Part model, mm, in its own coordinate system. Face numbers are marked on the shaded views. Coordinates: 2 decimals unless noted, no trailing zeros. Order: outer loops, then holes, each group sorted by start corner. A loop starts at its lowest first (then second) coordinate and runs counter-clockwise, first axis right, second up.
1) Mould opens along Z. For the marked faces 1, 2 and 3 say: +Z half, -Z half, draft (parallel to the pull), parting line (faces both ways), or undercut.
2) Cut at B-B (z = 11.25). List the corners of the cut face in (x, y), and give its area (3 significant figures).
3) Wall check: L1, parallel to Y at x = 8.3, z = 0.5; L2, parallel to Z at x = 8.75, y = 6.75; L3, parallel to Y at x = 7, z = 1.75. Give the ranges that are in metal, low to high.
4) Cut at C-C (y = 0). List the corners of the cut face in (x, z).
5) Cut at A-A (x = 8.3). List the corners of the cut face in (y, z).
6) Pin check, flat tips, straight feed: pin 1 Ø5 at (y, z) = (5.5, 2.5) entering from +X; pin 2 Ø0.5 at (y, z) = (4.5, 7) entering from +X; pin 3 Ø2 at (x, z) = (8, 3.5) entering from +Y; pin 4 Ø4.5 at (x, z) = (7.5, 5.5) entering from -Y. Stop position of each tip, or through.
7) Cut at D-D (x = 4.25). List the corners of the cut face in (y, z).
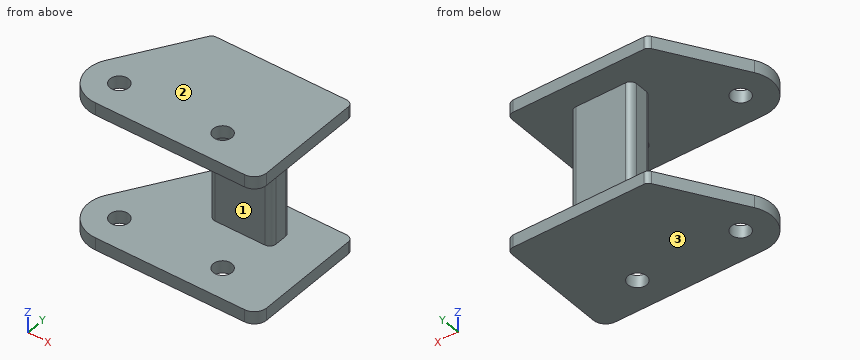
```python
from build123d import *

# Parameters (mm, degrees)
SKETCH1_R           = 0.75
BOSS_EXTRUDE1_DEPTH = 1
BOSS_EXTRUDE2_START = 1
BOSS_EXTRUDE2_DEPTH = 10
BOSS_EXTRUDE3_START = 11
SKETCH1_4_R         = 0.75
BOSS_EXTRUDE3_DEPTH = 1


with BuildPart() as part:
    # Sketch1 → Boss-Extrude1 (new body)
    with BuildSketch(Plane.XY):
        with BuildLine():
            Line((1.575471698, 7.264150943), (-2.122641509, 1.320754717))
            ThreePointArc((-2.122641509, 1.320754717), (-2.18539319, -1.214107328), (0, -2.5))
            Line((0, -2.5), (12, -2.5))
            ThreePointArc((12, -2.5), (12.707106781, -2.207106781), (13, -1.5))
            Line((13, -1.5), (13, 7))
            ThreePointArc((13, 7), (12.853553391, 7.353553391), (12.5, 7.5))
            Line((12.5, 7.5), (2, 7.5))
            ThreePointArc((2, 7.5), (1.757178534, 7.437078638), (1.575471698, 7.264150943))
        make_face()
        Circle(SKETCH1_R, mode=Mode.SUBTRACT)
        with Locations((8.3, 0)):
            Circle(SKETCH1_R, mode=Mode.SUBTRACT)
    extrude(amount=BOSS_EXTRUDE1_DEPTH)

    # Sketch1<3> → Boss-Extrude2 (add)
    with BuildSketch(Plane.XY.offset(BOSS_EXTRUDE2_START)):
        with BuildLine():
            Line((5, 5.5), (9, 5.5))
            ThreePointArc((9, 5.5), (9.353553391, 5.353553391), (9.5, 5))
            Line((9.5, 5), (9.5, 4))
            ThreePointArc((9.5, 4), (9.353553391, 3.646446609), (9, 3.5))
            Line((9, 3.5), (5, 3.5))
            ThreePointArc((5, 3.5), (4.646446609, 3.646446609), (4.5, 4))
            Line((4.5, 4), (4.5, 5))
            ThreePointArc((4.5, 5), (4.646446609, 5.353553391), (5, 5.5))
        make_face()
    extrude(amount=BOSS_EXTRUDE2_DEPTH)

    # Sketch1<4> → Boss-Extrude3 (add)
    with BuildSketch(Plane.XY.offset(BOSS_EXTRUDE3_START)):
        with BuildLine():
            Line((1.575471698, 7.264150943), (-2.122641509, 1.320754717))
            ThreePointArc((-2.122641509, 1.320754717), (-2.18539319, -1.214107328), (0, -2.5))
            Line((0, -2.5), (12, -2.5))
            ThreePointArc((12, -2.5), (12.707106781, -2.207106781), (13, -1.5))
            Line((13, -1.5), (13, 7))
            ThreePointArc((13, 7), (12.853553391, 7.353553391), (12.5, 7.5))
            Line((12.5, 7.5), (2, 7.5))
            ThreePointArc((2, 7.5), (1.757178534, 7.437078638), (1.575471698, 7.264150943))
        make_face()
        Circle(SKETCH1_4_R, mode=Mode.SUBTRACT)
        with Locations((8.3, 0)):
            Circle(SKETCH1_4_R, mode=Mode.SUBTRACT)
    extrude(amount=BOSS_EXTRUDE3_DEPTH)


solid = part.part
```
Geometry check:
1. face 1: undercut
1. face 2: +Z half
1. face 3: -Z half
2. outline: (-2.12, 1.32) arc R2.5 ccw to (0, -2.5) - (12, -2.5) arc R1 ccw to (13, -1.5) - (13, 7) arc R0.5 ccw to (12.5, 7.5) - (2, 7.5) arc R0.5 ccw to (1.58, 7.26) - close; hole circle Ø1.5 at (0, 0); hole circle Ø1.5 at (8.3, 0)
2. area: 135 mm2
3. L1: y = -2.5 to -0.75, 0.75 to 7.5
3. L2: z = 0 to 1, 11 to 12
3. L3: y = 3.5 to 5.5
4. outline: (-2.5, 0) - (-0.75, 0) - (-0.75, 1) - (-2.5, 1) - close; (-2.5, 11) - (-0.75, 11) - (-0.75, 12) - (-2.5, 12) - close; (0.75, 0) - (7.55, 0) - (7.55, 1) - (0.75, 1) - close; (0.75, 11) - (7.55, 11) - (7.55, 12) - (0.75, 12) - close; (9.05, 0) - (13, 0) - (13, 1) - (9.05, 1) - close; (9.05, 11) - (13, 11) - (13, 12) - (9.05, 12) - close
5. outline: (-2.5, 0) - (-0.75, 0) - (-0.75, 1) - (-2.5, 1) - close; (-2.5, 11) - (-0.75, 11) - (-0.75, 12) - (-2.5, 12) - close; (0.75, 0) - (7.5, 0) - (7.5, 1) - (5.5, 1) - (5.5, 11) - (7.5, 11) - (7.5, 12) - (0.75, 12) - (0.75, 11) - (3.5, 11) - (3.5, 1) - (0.75, 1) - close
6. pin 1: stops at x = 13
6. pin 2: stops at x = 9.5
6. pin 3: stops at y = 5.5
6. pin 4: stops at y = 3.5
7. outline: (-2.5, 0) - (7.5, 0) - (7.5, 1) - (-2.5, 1) - close; (-2.5, 11) - (7.5, 11) - (7.5, 12) - (-2.5, 12) - close
